```python
from build123d import *

# Parameters (mm, degrees)
SALIENTE_EXTRUIR1_DEPTH = 3
CORTAR_EXTRUIR3_DEPTH   = 10


with BuildPart() as part:
    # Croquis1 → Saliente-Extruir1 (new body)
    with BuildSketch(Plane.XY):
        Polygon((-99.368109251, 50.24258427), (-99.368109251, 31.74258427), (-96.368109251, 31.74258427), (-96.368109251, 10.74258427), (-99.368109251, 10.74258427), (-99.368109251, -10.25741573), (-96.368109251, -10.25741573), (-96.368109251, -31.25741573), (-99.368109251, -31.25741573), (-99.368109251, -49.75741573), (-72.868109251, -49.75741573), (-72.868109251, -46.75741573), (-51.868109251, -46.75741573), (-51.868109251, -49.75741573), (-30.868109251, -49.75741573), (-30.868109251, -46.75741573), (-9.868109251, -46.75741573), (-9.868109251, -49.75741573), (11.131890749, -49.75741573), (11.131890749, -46.75741573), (32.131890749, -46.75741573), (32.131890749, -49.75741573), (53.131890749, -49.75741573), (53.131890749, -46.75741573), (72.868109251, -46.75741573), (72.868109251, -50.24258427), (93.868109251, -50.24258427), (99.368109251, -50.24258427), (99.368109251, -31.74258427), (96.368109251, -31.74258427), (96.368109251, -10.74258427), (99.368109251, -10.74258427), (99.368109251, 10.25741573), (96.368109251, 10.25741573), (96.368109251, 31.25741573), (100.631890749, 31.25741573), (100.631890749, 50.24258427), (74.131890749, 50.24258427), (74.131890749, 47.24258427), (53.131890749, 47.24258427), (53.131890749, 50.24258427), (32.131890749, 50.24258427), (32.131890749, 47.24258427), (11.131890749, 47.24258427), (11.131890749, 50.24258427), (-9.868109251, 50.24258427), (-9.868109251, 47.24258427), (-30.868109251, 47.24258427), (-30.868109251, 50.24258427), (-51.868109251, 50.24258427), (-51.868109251, 47.24258427), (-72.868109251, 47.24258427), (-72.868109251, 50.24258427), (-93.868109251, 50.24258427), align=None)
    extrude(amount=SALIENTE_EXTRUIR1_DEPTH)

    # Croquis2 → Cortar-Extruir3 (cut)
    with BuildSketch(Plane.XY.offset(3)):
        Polygon((-72.868109251, 50.24258427), (-99.368109251, 50.24258427), (-99.368109251, 31.74258427), (-96.368109251, 31.74258427), (-96.368109251, 10.74258427), (-99.368109251, 10.74258427), (-99.368109251, -10.25741573), (-96.368109251, -10.25741573), (-96.368109251, -31.25741573), (-99.368109251, -31.25741573), (-99.368109251, -49.75741573), (-72.868109251, -49.75741573), (-72.868109251, -46.75741573), (-59.368109251, -46.75741573), (-59.368109251, 47.24258427), (-72.868109251, 47.24258427), align=None)
    extrude(amount=-CORTAR_EXTRUIR3_DEPTH, mode=Mode.SUBTRACT)


solid = part.part
```
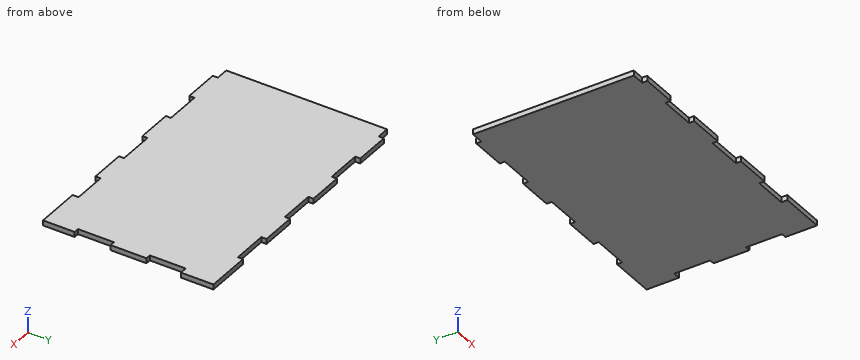
The listing builds one solid part. Answer for the finished solid, in the listing's coordinates (mm). Give positions to 0.01 mm unless a question says otherwise; leave off trailing zeros. Order: outer loops, then holes, each group sorted by start corner. A loop starts at its lowest first (then second) coordinate and runs counter-clockwise, first axis right, second up.
Item 1: The part is cut by section B-B, the plane x = -23. Give the vertices of the cut face in (y, z), and give its area (3 significant figures).
From the geometry:
outline: (-46.76, 0) - (47.24, 0) - (47.24, 3) - (-46.76, 3) - close
area: 282 mm2
Item 2: The part is cut by section A-A, the plane y = -28.5. Give the vertices of the cut face in (x, z).
From the geometry:
outline: (-59.37, 0) - (96.37, 0) - (96.37, 3) - (-59.37, 3) - close
Item 3: Given pin 1 Ø0.9 at (y, z) = (48.5, 1) entering from -X; pin 2 Ø0.9 at (y, z) = (-18.5, 1.5) entering from +X; pin 3 Ø0.9 at (y, z) = (-48.5, 1.5) entering from +X, each flat-ended and moving along its own axis, determine where each tip first touches the part or whether it passes through.
From the geometry:
pin 1: stops at x = -51.87
pin 2: stops at x = 96.37
pin 3: stops at x = 99.37
Item 4: Find the intervals of material crossed by probe 1 along Y at (x, z) = (45.5, 2.3); probe 2 along Y at (x, z) = (66, 0.95); probe 3 along X at (y, z) = (23, 0.9), in increasing order.
From the geometry:
probe 1: y = -49.76 to 50.24
probe 2: y = -46.76 to 47.24
probe 3: x = -59.37 to 96.37
